Part model, mm, in its own coordinate system. A direction names the side the tool comes from. Give positions to 0.01 mm unless a question says otherwise; leave off trailing zeros. Write each loop counter-clockwise with the first axis right and the second up, starting at its lowest first coordinate (ties: lowest second). Pieces come first, ordered by that corner, then holes. Notation, with made-up numbers: M 34.25,83 L 91.25,83 A22 cw 91.25,100 Z; hole C 85.25,66.25 d6. An arc over 180 degrees is marked long. Use CSV: the item, a comma, the result in double quotes. Start each with the question number.
Item 1: Cut at C-C (y = 62). List the corners of the cut face in (x, z), then the cut area to 3 significant figures.
Item 2: Mould opens along Z. For faces 1 (the flat face through (3, 90, -29)), 2 (the cylindrical face through (2, 119, -1)), 3 (the cylindrical face through (13.04, 8.52, 8.66)), 4 (the cylindrical face through (3.042, 88.289, -9.804)) say: released by +Z, released by -Z, zero draft, split by the parting line, or undercut.
Item 3: Pin check, flat tips, straight feed: pin 1 (7 mm diameter, centred on y = 155, z = -23.5, fed in from +X); pin 2 (3 mm diameter, centred on x = 5, z = -10, fed in from -Y); pin 3 (3 mm diameter, centred on y = 188.5, z = -19.5, fed in from +X). Stop position of each tip, or through.
Item 4: Drill centre lines: line 1 (Y direction, x = 5, z = -23); line 2 (Y direction, x = 0.95, z = -23.5); line 3 (Y direction, x = 13.7, z = 17). Where is each one in solid material? Low to high. Write a range as [from, to].
Item 5: Which spindle directions (+Z, -Z, +X, -X, +Y, -Y) get a long thin tool onto all of the face, cutting with end or side? Do faces 5 (the flat face through (22, 110, 6)), 6 (the flat face through (3, 41, -8)), 7 (the flat face through (2, 153, -25)), 8 (the flat face through (10, 116, -6)). Say none if no direction does.
Item 6: Cut at A-A (y = 175). List the corners of the cut face in (x, z), then the cut area to 3 significant figures.
Item 7: Cut at B-B (y = 7). List the corners of the cut face in (x, z), then the cut area to 3 significant figures.
Item 8: Cut at D-D (x = 14). List the corners of the cut face in (y, z), then the cut area to 3 significant figures.
from build123d import *

# Parameters (mm, degrees)
SCHIZZO1_W                                           = 235
SCHIZZO1_H                                           = 65
ESTRUSIONE_ESTRUSIONE1_DEPTH                         = 16
SCHIZZO2_W                                           = 10
SCHIZZO2_H                                           = 37
TAGLIO_ESTRUSIONE1_DEPTH                             = 240.436839271
SCHIZZO3_W                                           = 35
SCHIZZO3_H                                           = 90
TAGLIO_ESTRUSIONE2_DEPTH                             = 240.436839271
SCHIZZO4_W                                           = 10
SCHIZZO4_H                                           = 22
TAGLIO_ESTRUSIONE3_DEPTH                             = 240.436839271
FORO_LAMATO_PER_VITE_M4_A_TESTA_ESAGONAL_D           = 4.5
FORO_LAMATO_PER_VITE_M4_A_TESTA_ESAGONAL_CBORE_D     = 8
FORO_LAMATO_PER_VITE_M4_A_TESTA_ESAGONAL_CBORE_DEPTH = 4
RACCORDO1_R                                          = 2
RACCORDO2_R                                          = 4
RACCORDO3_R                                          = 5
RACCORDO4_R                                          = 6
FORO_PER_VITE_M4_1_D                                 = 4.5
FORO_PER_VITE_M4_1_DEPTH                             = 188
FORO_PER_VITE_M4_1_TIP                               = 1.351936393
SCHIZZO9_W                                           = 3
SCHIZZO9_H                                           = 15
ESTRUSIONE_ESTRUSIONE2_DEPTH                         = 15
SCHIZZO10_R                                          = 3
TAGLIO_ESTRUSIONE4_DEPTH                             = 15
SMUSSO1_SIZE                                         = 8


with BuildPart() as part:
    # Schizzo1 → Estrusione-Estrusione1 (new body)
    with BuildSketch(Plane(origin=(0, 0, 0), x_dir=(0, -1, 0), z_dir=(-1, 0, 0))):
        with Locations((-117.5, -10.5)):
            Rectangle(SCHIZZO1_W, SCHIZZO1_H)
    extrude(amount=-ESTRUSIONE_ESTRUSIONE1_DEPTH)

    # Schizzo2 → Taglio-Estrusione1 (cut, through all)
    with BuildSketch(Plane.XZ):
        with Locations((11, -24.5)):
            Rectangle(SCHIZZO2_W, SCHIZZO2_H)
    extrude(amount=-TAGLIO_ESTRUSIONE1_DEPTH, mode=Mode.SUBTRACT)

    # Schizzo3 → Taglio-Estrusione2 (cut, through all)
    with BuildSketch(Plane.ZY):
        with Locations((-25.5, 45)):
            Rectangle(SCHIZZO3_W, SCHIZZO3_H)
    extrude(amount=-TAGLIO_ESTRUSIONE2_DEPTH, mode=Mode.SUBTRACT)

    # Schizzo4 → Taglio-Estrusione3 (cut, through all)
    with BuildSketch(Plane.XZ):
        with Locations((5, 11)):
            Rectangle(SCHIZZO4_W, SCHIZZO4_H)
    extrude(amount=-TAGLIO_ESTRUSIONE3_DEPTH, mode=Mode.SUBTRACT)

    # Foro lamato per Vite M4 a testa esagonale-1 (through all)
    with Locations(Plane(origin=(6, 0, 0), x_dir=(0, 0, -1), z_dir=(1, 0, 0))):
        with Locations((23.5, 175), (23.5, 155), (23.5, 135)):
            CounterBoreHole(FORO_LAMATO_PER_VITE_M4_A_TESTA_ESAGONAL_D / 2, FORO_LAMATO_PER_VITE_M4_A_TESTA_ESAGONAL_CBORE_D / 2, FORO_LAMATO_PER_VITE_M4_A_TESTA_ESAGONAL_CBORE_DEPTH)

    # Raccordo1
    raccordo1_edges = [part.edges().sort_by_distance(p)[0] for p in [
        (10, 117.5, 0),
        (6, 117.5, -6),
    ]]
    fillet(raccordo1_edges, radius=RACCORDO1_R)

    # Raccordo2
    raccordo2_edges = [part.edges().sort_by_distance(p)[0] for p in [
        (16, 117.5, -6),
    ]]
    fillet(raccordo2_edges, radius=RACCORDO2_R)

    # Raccordo3
    raccordo3_edges = [part.edges().sort_by_distance(p)[0] for p in [
        (0, 117.5, 0),
    ]]
    fillet(raccordo3_edges, radius=RACCORDO3_R)

    # Raccordo4
    raccordo4_edges = [part.edges().sort_by_distance(p)[0] for p in [
        (3, 90, -8),
    ]]
    fillet(raccordo4_edges, radius=RACCORDO4_R)

    # Foro per Vite M4-1
    with Locations(Plane.ZY.offset(-10)):
        with Locations((17, 7), (7, 7)):
            Hole(FORO_PER_VITE_M4_1_D / 2, depth=FORO_PER_VITE_M4_1_DEPTH)
            with Locations((0, 0, -(FORO_PER_VITE_M4_1_DEPTH + FORO_PER_VITE_M4_1_TIP / 2))):  # 118° drill point
                Cone(0, FORO_PER_VITE_M4_1_D / 2, FORO_PER_VITE_M4_1_TIP, mode=Mode.SUBTRACT)

    # Schizzo9 → Estrusione-Estrusione2 (add)
    with BuildSketch(Plane(origin=(16, 0, 0), x_dir=(0, 0, -1), z_dir=(1, 0, 0))):
        with Locations((-7.5, 117.5)):
            Rectangle(SCHIZZO9_W, SCHIZZO9_H)
    extrude(amount=ESTRUSIONE_ESTRUSIONE2_DEPTH)

    # Schizzo10 → Taglio-Estrusione4 (cut)
    with BuildSketch(Plane(origin=(16, 0, 0), x_dir=(0, 0, -1), z_dir=(1, 0, 0))):
        with Locations((-13, 117.5)):
            Circle(SCHIZZO10_R)
    extrude(amount=-TAGLIO_ESTRUSIONE4_DEPTH, mode=Mode.SUBTRACT)

    # Smusso1
    smusso1_edges = [part.edges().sort_by_distance(p)[0] for p in [
        (16, 117.5, 6),
    ]]
    chamfer(smusso1_edges, length=SMUSSO1_SIZE - 0.0001)  # a hair under: the kernel refuses the full size


solid = part.part
Worked answers:
1,outline,"M 0,-8 L 6,-8 A2 cw 8,-6 L 12,-6 A4 ccw 16,-2 L 16,22 L 10,22 L 10,2 A2 cw 8,0 L 5,0 A5 ccw 0,-5 Z"
1,area,"233 mm^2"
2,face 1,"zero draft"
2,face 2,"released by +Z"
2,face 3,"undercut"
2,face 4,"released by -Z"
3,pin 1,"stops at x = 2"
3,pin 2,"stops at y = 86.4"
3,pin 3,"stops at x = 6"
4,line 1,"y = [90, 131.03], [138.97, 151.03], [158.97, 171.03], [178.97, 235]"
4,line 2,"y = [90, 132.75], [137.25, 152.75], [157.25, 172.75], [177.25, 235]"
4,line 3,"y = [0, 4.75], [9.25, 235]"
5,face 5,"+Z, -Z, +X, -Y"
5,face 6,"-Z, +X, -X, -Y"
5,face 7,"+X"
5,face 8,"-Z, +X, +Y, -Y"
6,outline,"M 0,-43 L 6,-43 L 6,-27.5 L 2,-27.5 L 2,-25.75 L 0,-25.75 Z; M 0,-21.25 L 2,-21.25 L 2,-19.5 L 6,-19.5 L 6,-8 A2 cw 8,-6 L 12,-6 A4 ccw 16,-2 L 16,22 L 10,22 L 10,2 A2 cw 8,0 L 5,0 A5 ccw 0,-5 Z"
6,area,"402 mm^2"
7,outline,"M 0,-8 L 6,-8 A2 cw 8,-6 L 12,-6 A4 ccw 16,-2 L 16,4.75 L 10,4.75 L 10,2 A2 cw 8,0 L 5,0 A5 ccw 0,-5 Z; M 10,9.25 L 16,9.25 L 16,14.75 L 10,14.75 Z; M 10,19.25 L 16,19.25 L 16,22 L 10,22 Z"
7,area,"179 mm^2"
8,outline,"M 0,-5.46 L 235,-5.46 L 235,22 L 0,22 Z; hole C 7,7 d4.5; hole C 7,17 d4.5; hole C 117.5,13 d6"
8,area,"6,390 mm^2"
